from build123d import *

# Parameters (mm, degrees)
SKETCH2_R           = 7.5
BOSS_EXTRUDE1_DEPTH = 100
SKETCH3_R           = 12.5
BOSS_EXTRUDE2_DEPTH = 5
BOSS_EXTRUDE3_START = 5
SKETCH4_R           = 12.5
BOSS_EXTRUDE3_DEPTH = 5
SCALE1_SCALE        = 0.5


with BuildPart() as part:
    # Sketch2 → Boss-Extrude1 (new body)
    with BuildSketch(Plane(origin=(0, 0, 0), x_dir=(1, 0, 0), z_dir=(0, 1, 0))):
        with Locations(Location((0, 0, 0), (0, 0, 270))):
            Circle(SKETCH2_R)
    extrude(amount=BOSS_EXTRUDE1_DEPTH)

    # Sketch3 → Boss-Extrude2 (add)
    with BuildSketch(Plane(origin=(0, 100, 0), x_dir=(1, 0, 0), z_dir=(0, 1, 0))):
        with Locations(Location((0, 0, 0), (0, 0, 270))):
            Circle(SKETCH3_R)
    extrude(amount=BOSS_EXTRUDE2_DEPTH)

    # Sketch4 → Boss-Extrude3 (add)
    with BuildSketch(Plane.XZ.offset(BOSS_EXTRUDE3_START)):
        with Locations(Location((0, 0, 0), (0, 0, 90))):
            Circle(SKETCH4_R)
    extrude(amount=-BOSS_EXTRUDE3_DEPTH)


with BuildPart() as part_1:
    # Scale1: scaled about (0, 50, 0)
    add(part.part.scale(SCALE1_SCALE).moved(Location((0, 25, 0))))


solid = part_1.part
Model file for the job. Use its own axes, mm. A direction names the side the tool comes from. Round coordinates to 2 decimals unless told otherwise and drop trailing zeros. Loops run counter-clockwise (first coordinate to the right, second up) from the corner with the lowest first, then second, coordinate; pieces in that order, holes last. Notation, with made-up numbers: M -34.5,-2 L -24.5,-2 A17 cw -24.5,2 Z; hole C 3,22.25 d11. An arc over 180 degrees is marked long. One line per question, with ' | ' between items.
1) Band-saw the part on D-D (y = 52.5). Give the cut face in (x, z).
Solved:
outline: C 0,0 d7.5
2) Flat gauge pins, fed straight in: pin 1 (6 mm diameter, centred on y = 41, z = 0.5, fed in from -X); pin 2 (1.5 mm diameter, centred on x = -3.5, y = 36.5, fed in from -Z); pin 3 (2 mm diameter, centred on y = 52.5, z = 0, fed in from +X). Where does each tip first touch, or does it go through?
Solved:
pin 1: stops at x = -3.75 | pin 2: stops at z = -2.55 | pin 3: stops at x = 3.75
3) Band-saw the part on C-C (x = 0). Give the cut face in (y, z), then the cut area to 4 significant figures.
Solved:
outline: M 22.5,-6.25 L 25,-6.25 L 25,-3.75 L 75,-3.75 L 75,-6.25 L 77.5,-6.25 L 77.5,6.25 L 75,6.25 L 75,3.75 L 25,3.75 L 25,6.25 L 22.5,6.25 Z | area: 437.5 mm²
4) Band-saw the part on A-A (z = -5.5). Give the cut face in (x, y).
Solved:
outline: M -2.97,22.5 L 2.97,22.5 L 2.97,25 L -2.97,25 Z; M -2.97,75 L 2.97,75 L 2.97,77.5 L -2.97,77.5 Z
5) 3-axis set-ups, long thin cutter, end or side, ignore diameter. For faces 1 (the flat face through (0, 77.5, 0)), 2 (the flat face through (-3, 75, 3)): which of +Z, -Z, +X, -X, +Y, -Y reach the whole face in a straight line?
Solved:
face 1: +Z, -Z, +X, -X, +Y | face 2: none
6) Band-saw the part on B-B (z = 0). Give the cut face in (x, y), then the cut area to 4 significant figures.
Solved:
outline: M -6.25,22.5 L 6.25,22.5 L 6.25,25 L 3.75,25 L 3.75,75 L 6.25,75 L 6.25,77.5 L -6.25,77.5 L -6.25,75 L -3.75,75 L -3.75,25 L -6.25,25 Z | area: 437.5 mm²
7) Drill centre lines: line 1 along Y through (x, z) = (2.5, -3.25); line 2 along X through (y, z) = (31, -2); line 3 along Z through (x, y) = (1, 52.5). Where is each one in solid material? Low to high.
Solved:
line 1: y = 22.5 to 25, 75 to 77.5 | line 2: x = -3.17 to 3.17 | line 3: z = -3.61 to 3.61
8) Mould opens along Y. For faces 3 (the cylindrical face through (1.88, 76.23, 5.96)), 4 (the flat face through (0, 22.5, 0)), 5 (the cylindrical face through (0.165, 49.65, -3.746)) say: +Y half, -Y half, draft (parallel to the pull), parting line (faces both ways), or undercut.
Solved:
face 3: draft | face 4: -Y half | face 5: undercut
